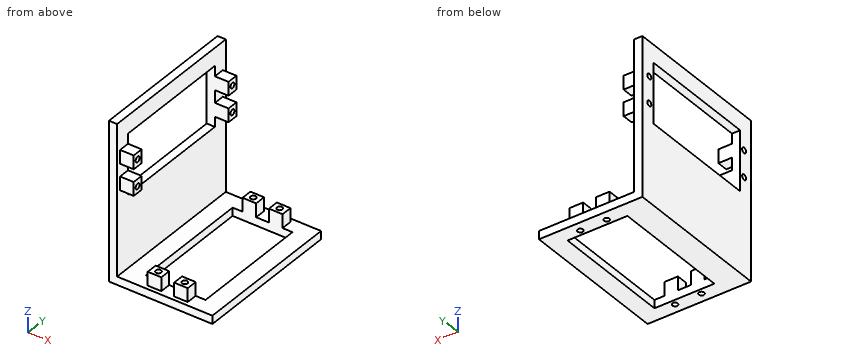
from build123d import *

# Parameters (mm, degrees)
BOSS_EXTRUDE1_DEPTH = 27.5
SKETCH3_R           = 1
SKETCH3_W           = 22
SKETCH3_H           = 44
CUT_EXTRUDE1_DEPTH  = 3
SKETCH4_R           = 1
SKETCH4_W           = 22
SKETCH4_H           = 44
CUT_EXTRUDE2_DEPTH  = 3
SKETCH5_W           = 5
SKETCH5_H           = 4
BOSS_EXTRUDE2_DEPTH = 5
CUT_EXTRUDE3_START  = -5
SKETCH6_R           = 1
CUT_EXTRUDE3_DEPTH  = 5
BOSS_EXTRUDE3_START = 5
SKETCH7_W           = 5
SKETCH7_H           = 4
SKETCH7_R           = 1
BOSS_EXTRUDE3_DEPTH = 5


with BuildPart() as part:
    # Sketch1 → Boss-Extrude1 (new, symmetric)
    with BuildSketch(Plane(origin=(0, 0, 0), x_dir=(1, 0, 0), z_dir=(0, 1, 0))):
        Polygon((38, 0), (0, 0), (0, -58), (3, -58), (3, -3), (38, -3), align=None)
    extrude(amount=BOSS_EXTRUDE1_DEPTH, both=True)

    # Sketch3 → Cut-Extrude1 (cut)
    with BuildSketch(Plane.XY.offset(3)):
        with Locations((15.65, -24)):
            Circle(SKETCH3_R)
        with Locations((25.35, -24)):
            Circle(SKETCH3_R)
        with Locations((25.35, 24)):
            Circle(SKETCH3_R)
        with Locations((15.65, 24)):
            Circle(SKETCH3_R)
        with Locations((20.5, 0)):
            Rectangle(SKETCH3_W, SKETCH3_H)
    extrude(amount=-CUT_EXTRUDE1_DEPTH, mode=Mode.SUBTRACT)

    # Sketch4 → Cut-Extrude2 (cut)
    with BuildSketch(Plane(origin=(3, 0, 0), x_dir=(0, 0, -1), z_dir=(1, 0, 0))):
        with Locations((-45.35, -24)):
            Circle(SKETCH4_R)
        with Locations((-35.65, -24)):
            Circle(SKETCH4_R)
        with Locations((-35.65, 24)):
            Circle(SKETCH4_R)
        with Locations((-45.35, 24)):
            Circle(SKETCH4_R)
        with Locations((-40.5, 0)):
            Rectangle(SKETCH4_W, SKETCH4_H)
    extrude(amount=-CUT_EXTRUDE2_DEPTH, mode=Mode.SUBTRACT)

    # Sketch5 → Boss-Extrude2 (add)
    with BuildSketch(Plane(origin=(3, 0, 0), x_dir=(0, 0, -1), z_dir=(1, 0, 0))):
        with Locations((-45.35, -24)):
            Rectangle(SKETCH5_W, SKETCH5_H)
        with Locations((-35.765327537, -24)):
            Rectangle(SKETCH5_W, SKETCH5_H)
        with Locations((-35.65, 24)):
            Rectangle(SKETCH5_W, SKETCH5_H)
        with Locations((-45.234672463, 24)):
            Rectangle(SKETCH5_W, SKETCH5_H)
    extrude(amount=BOSS_EXTRUDE2_DEPTH)

    # Sketch6 → Cut-Extrude3 (cut)
    with BuildSketch(Plane.ZY.offset(-3).offset(CUT_EXTRUDE3_START)):
        with Locations(Location((35.65, -24, 0), (0, 0, 180))):
            Circle(SKETCH6_R)
        with Locations(Location((45.35, -24, 0), (0, 0, 180))):
            Circle(SKETCH6_R)
        with Locations(Location((45.35, 24, 0), (0, 0, 180))):
            Circle(SKETCH6_R)
        with Locations(Location((35.65, 24, 0), (0, 0, 180))):
            Circle(SKETCH6_R)
    extrude(amount=CUT_EXTRUDE3_DEPTH, mode=Mode.SUBTRACT)

    # Sketch7 → Boss-Extrude3 (add)
    # profile 1 of 4: a face of its own
    with BuildSketch(Plane.XY.offset(3).offset(BOSS_EXTRUDE3_START)):
        with Locations((15.65, -24)):
            Rectangle(SKETCH7_W, SKETCH7_H)
        with Locations((15.65, -24)):
            Circle(SKETCH7_R, mode=Mode.SUBTRACT)
    # profile 2 of 4: a face of its own
    with BuildSketch(Plane.XY.offset(3).offset(BOSS_EXTRUDE3_START)):
        with Locations((25.35, -24)):
            Rectangle(SKETCH7_W, SKETCH7_H)
        with Locations((25.35, -24)):
            Circle(SKETCH7_R, mode=Mode.SUBTRACT)
    # profile 3 of 4: a face of its own
    with BuildSketch(Plane.XY.offset(3).offset(BOSS_EXTRUDE3_START)):
        with Locations((25.35, 24)):
            Rectangle(SKETCH7_W, SKETCH7_H)
        with Locations((25.35, 24)):
            Circle(SKETCH7_R, mode=Mode.SUBTRACT)
    # profile 4 of 4: a face of its own
    with BuildSketch(Plane.XY.offset(3).offset(BOSS_EXTRUDE3_START)):
        with Locations((15.65, 24)):
            Rectangle(SKETCH7_W, SKETCH7_H)
        with Locations((15.65, 24)):
            Circle(SKETCH7_R, mode=Mode.SUBTRACT)
    extrude(amount=-BOSS_EXTRUDE3_DEPTH)


solid = part.part
Here's how the part is built. I have some questions about the finished solid (model axes, mm). Round coordinates to 2 decimals unless told otherwise and drop trailing zeros. Order: outer loops, then holes, each group sorted by start corner. A loop starts at its lowest first (then second) coordinate and runs counter-clockwise, first axis right, second up. Notation, with made-up numbers: (51, 50.5) -> (81, 50.5) arc R20 cw to (81, 61.5) -> close; hole circle Ø7 at (41.5, 5). An arc over 180 degrees is marked (long way). Use CSV: the item, a comma, the result in double quotes.
1. I need wall thicknesses on line 1 along Z through (x, y) = (4, -24); line 2 along Y through (x, z) = (25.35, 1.5); line 3 along Z through (x, y) = (5.5, 24). Which ranges of each line are inside material? Lowest first, please.
Recorded:
line 1,"z = 0 to 3, 33.27 to 34.65, 36.65 to 38.27, 42.85 to 44.35, 46.35 to 47.85"
line 2,"y = -27.5 to -25, -23 to -22, 22 to 23, 25 to 27.5"
line 3,"z = 0 to 3, 33.15 to 34.65, 36.65 to 38.15, 42.73 to 44.35, 46.35 to 47.73"
2. I want a section at B-B on z = 50. List the corners of the cut face in (x, y) for me.
Recorded:
outline,"(0, -27.5) -> (3, -27.5) -> (3, -22) -> (0, -22) -> close; (0, 22) -> (3, 22) -> (3, 27.5) -> (0, 27.5) -> close"
3. I'm going to push flat-ended pins straight in: P1, Ø10, axis at y = 21, z = 40.5, coming from the +X side; P2, Ø8, axis at y = -14, z = 21.5, coming from the +X side; P3, Ø10, axis at x = 30.5, y = -14.5, coming from the +Z side. Where does each tip first touch, or does it pass through?
Recorded:
P1,"stops at x = 8"
P2,"stops at x = 3"
P3,"stops at z = 3"
4. I want a section at A-A on x = 5. Give the number of separate pieces and of enclosed holes in the cut face, and give its area (3 significant figures).
Recorded:
separate pieces,"5"
enclosed holes,"4"
area,"232 mm2"
5. I want a section at C-C on x = 25.35. List the corners of the cut face in (y, z) for me, and give its area (3 significant figures).
Recorded:
outline,"(-27.5, 0) -> (-25, 0) -> (-25, 8) -> (-26, 8) -> (-26, 3) -> (-27.5, 3) -> close; (-23, 0) -> (-22, 0) -> (-22, 8) -> (-23, 8) -> close; (22, 0) -> (23, 0) -> (23, 8) -> (22, 8) -> close; (25, 0) -> (27.5, 0) -> (27.5, 3) -> (26, 3) -> (26, 8) -> (25, 8) -> close"
area,"41.0 mm2"
6. I want a section at D-D on y = 19. List the corners of the cut face in (x, z) for me, and give its area (3 significant figures).
Recorded:
outline,"(0, 0) -> (9.5, 0) -> (9.5, 3) -> (3, 3) -> (3, 29.5) -> (0, 29.5) -> close; (0, 51.5) -> (3, 51.5) -> (3, 58) -> (0, 58) -> close; (31.5, 0) -> (38, 0) -> (38, 3) -> (31.5, 3) -> close"
area,"147 mm2"
